Autodesk Inventor part; units mm, degrees
ref_plane "Work Plane2" through (-1200, 0, -1300) normal (0, 0, 1) x (1, 0, 0)
ref_plane "Work Plane3" through (-600, 0, -2600) normal (-1, 0, 0) x (0, 0, 1)
ref_plane "YZ Plane" through (0, 0, 0) normal (1, 0, 0) x (0, 1, 0)
sketch "Sketch1" plane through (0, 0, 0) normal (0, 1, 0) x (-1, 0, 0)
  line L0 (0, 0) -> (1200, 0)
  line L1 (1200, 0) -> (1200, -2600)
  line L2 (1200, -2600) -> (0, -2600)
  line L3 (0, -2600) -> (0, 0)
  dimension "d0" = 1200
  dimension "d1" = 2600
extrude "Extrusion1" add sketch "Sketch1" along normal blind 50
sketch "Sketch2" plane through (0, 0, 0) normal (1, 0, 0) x (0, 0, -1)
  circle A0 centre (150, 25) radius 4.25
  line L0 (2600, 0) -> (0, 0)
  line L1 (0, 0) -> (0, 50)
  dimension "d4" = 8.5
  dimension "d5" = 25
  dimension "d8" = 150
extrude "Extrusion2" cut sketch "Sketch2" against normal blind 10
ref_plane "Work Plane2" through (-1200, 0, -1300) normal (0, 0, 1) x (1, 0, 0)
ref_plane "Work Plane3" through (-600, 0, -2600) normal (-1, 0, 0) x (0, 0, 1)
mirror "Mirror1" about plane through (-1200, 0, -1300) normal (0, 0, 1) of "Extrusion2"
mirror "Mirror2" about plane through (-600, 0, -2600) normal (-1, 0, 0) of "Extrusion2", "Mirror1"
properties part number "InsulatorWallNorrowasa" material "Polyethylene, Low Density"
Source: CAD feature listing. Evaluate the final solid. Frame: model axes, mm. Round coordinates to 2 decimals unless told otherwise and drop trailing zeros. One line per item, written item: value. Start each with the question number.
Item 1: Pin query (flat end, axial travel): pin 1 (5 mm diameter, centred on y = 25, z = -150, fed in from -X); pin 2 (2 mm diameter, centred on y = 11, z = -936, fed in from +X); pin 3 (2.5 mm diameter, centred on y = 25, z = -151, fed in from +X). Return the tip coordinate at first contact, or that it passes through.
Item 2: Ray query, L1, parallel to Y at x = -2.75, z = -150. Return the intervals inside material, ascending. Write a range as from..to.
Item 3: Mould query, pull axis Z, two halves, no side actions, for faces 1 (the flat face through (-592, 25, 0)), 2 (the flat face through (-592, 0, -1282)), 3 (the flat face through (-608, 25, -2600)). Classes: pulls with the +Z half, pulls with the -Z half, needs draft (parallel to the pull), parting line crosses it, or undercut.
Result set:
1. pin 1: stops at x = -1190
1. pin 2: stops at x = 0
1. pin 3: stops at x = -10
2. L1: y = 0..20.75, 29.25..50
3. face 1: pulls with the +Z half
3. face 2: needs draft
3. face 3: pulls with the -Z half
